from build123d import *

# Parameters (mm, degrees)
F0_W     = 75
F0_H     = 100
F0_R     = 4
F1_DEPTH = 2
F2_R     = 1.5
F2_W     = 18
F2_H     = 18
F3_DEPTH = 1


with BuildPart() as f1:
    # F0 (on Top) → F1 (new body)
    with BuildSketch(Plane.XY):
        Rectangle(F0_W, F0_H)
        with Locations((-28.5, -41)):
            Circle(F0_R, mode=Mode.SUBTRACT)
        with Locations((-28.5, 41)):
            Circle(F0_R, mode=Mode.SUBTRACT)
    extrude(amount=F1_DEPTH)

    # F2 (on face) → F3 (join)
    with BuildSketch(Plane.XY.offset(2)):
        with Locations((-19.536053, 35.5)):
            Circle(F2_R)
        with Locations((-15.603451, 35.5)):
            Circle(F2_R)
        with Locations((-15.603451, 40)):
            Circle(F2_R)
        with Locations((-4.571911, 40.951985)):
            Circle(F2_R)
        with Locations((-4.21, 35.965101)):
            Circle(F2_R)
        with Locations((0, 35.5)):
            Circle(F2_R)
        with Locations((-19.647178, 31.842151)):
            Circle(F2_R)
        with Locations((7.212908, 39.913771)):
            Circle(F2_R)
        with Locations((10.297806, 35.5)):
            Circle(F2_R)
        with Locations((30.034842, 22.869634)):
            Circle(F2_R)
        with Locations((33.795666, 18.915948)):
            Circle(F2_R)
        with Locations((23.573941, 24.219673)):
            Circle(F2_R)
        with Locations((18.17378, 24.219673)):
            Circle(F2_R)
        with Locations((18.17378, 19.976692)):
            Circle(F2_R)
        with Locations((18.17378, 15.733711)):
            Circle(F2_R)
        with Locations((8.144919, 24.026811)):
            Circle(F2_R)
        with Locations((-2.288573, 20.540619)):
            Circle(F2_R)
        with Locations((-7.4712, 20.417223)):
            Circle(F2_R)
        with Locations((-7.594596, 24.242494)):
            Circle(F2_R)
        with Locations((-17.466265, 24.242494)):
            Circle(F2_R)
        with Locations((-23.265871, 20.664013)):
            Circle(F2_R)
        with Locations((-23.265871, 15.851575)):
            Circle(F2_R)
        with Locations((-23.30542, 7.768475)):
            Circle(F2_R)
        with Locations((-23.30542, 2.26867)):
            Circle(F2_R)
        with Locations((-14.643229, 5.981038)):
            Circle(F2_R)
        with Locations((-9.005929, 1.4437)):
            Circle(F2_R)
        with Locations((-13.268277, -3.231134)):
            Circle(F2_R)
        with Locations((1.856185, 5.981038)):
            Circle(F2_R)
        with Locations((7.355989, 1.4437)):
            Circle(F2_R)
        with Locations((1.168709, -4.743581)):
            Circle(F2_R)
        with Locations((17.393135, -6.668512)):
            Circle(F2_R)
        with Locations((17.805619, 5.981038)):
            Circle(F2_R)
        Polygon((18.085241, -16.139069), (6.80601, -32.65509), (27.931091, -33.547665), align=None)
        with Locations((-9, -23.65509)):
            Rectangle(F2_W, F2_H)
    extrude(amount=F3_DEPTH)


solid = f1.part
Could you check a few things on this model? Use its own coordinates, in mm. A direction names the side the tool comes from. Coordinates: 2 decimals unless noted, no trailing zeros. Order: outer loops, then holes, each group sorted by start corner. A loop starts at its lowest first (then second) coordinate and runs counter-clockwise, first axis right, second up.
Q1. Suppose I cut it at A-A on y = -41. Please give me the cut outline in (x, z).
Q2. Suppose I cut it at C-C on x = 23.5. Please give me the cut outline in (y, z), and give its area (3 significant figures).
Q3. Will these pins go through, and if not, where does the flat tip stop? pin 1 (10.5 mm diameter, centred on x = -28.5, y = 41, fed in from -Z); pin 2 (0.8 mm diameter, centred on y = -24, z = 2.5, fed in from -X); pin 3 (3 mm diameter, centred on x = -21, y = -27.5, fed in from +Z); pin 4 (0.8 mm diameter, centred on x = -8.5, z = 2.5, fed in from -Y).
Q4. Suppose I cut it at B-B on x = -28.5. Please give me the cut outline in (y, z).
Q5. Thinking about a two-plate mould opening in Y: for faces 3 (the flat face through (10, 36, 3)), 4 (the cylindrical face through (-29.021, -37.034, 0.986)), which applies, released by +Y, released by -Y, zero draft, split by the parting line, or undercut?
Q6. Suppose I cut it at D-D on y = -31. Please give me the cut outline in (x, z), and give its area (3 significant figures).
Q7. Please list where these lines run through material, in increasing order: L1, parallel to Y at x = -28.5, z = 1; L2, parallel to Y at x = -23.5, z = 2.05; L3, parallel to Y at x = -8, z = 2.3.
Q8. Which directions (+Z, -Z, +X, -X, +Y, -Y) give clear straight access to the entire face, cutting with the end or side of a thin tool? Please do faces 1 (the flat face through (17, -27, 3)), 2 (the cylindrical face through (25.005, 24.67, 2.493)).
Answer:
1. outline: (-37.5, 0) - (-32.5, 0) - (-32.5, 2) - (-37.5, 2) - close; (-24.5, 0) - (37.5, 0) - (37.5, 2) - (-24.5, 2) - close
2. outline: (-50, 0) - (50, 0) - (50, 2) - (25.72, 2) - (25.72, 3) - (22.72, 3) - (22.72, 2) - (-25.71, 2) - (-25.71, 3) - (-33.36, 3) - (-33.36, 2) - (-50, 2) - close
2. area: 211 mm2
3. pin 1: stops at z = 0
3. pin 2: stops at x = -18
3. pin 3: stops at z = 2
3. pin 4: stops at y = -32.66
4. outline: (-50, 0) - (-45, 0) - (-45, 2) - (-50, 2) - close; (-37, 0) - (37, 0) - (37, 2) - (-37, 2) - close; (45, 0) - (50, 0) - (50, 2) - (45, 2) - close
5. face 3: zero draft
5. face 4: undercut
6. outline: (-37.5, 0) - (37.5, 0) - (37.5, 2) - (26.49, 2) - (26.49, 3) - (7.94, 3) - (7.94, 2) - (0, 2) - (0, 3) - (-18, 3) - (-18, 2) - (-37.5, 2) - close
6. area: 187 mm2
7. L1: y = -50 to -45, -37 to 37, 45 to 50
7. L2: y = 0.78 to 3.76, 6.28 to 9.26, 14.37 to 17.33, 19.18 to 22.15
7. L3: y = -32.66 to -14.66, 0.33 to 2.56, 19.01 to 21.82, 22.8 to 25.69
8. face 1: +Z, +X, -X, +Y, -Y
8. face 2: +Z
